```python
from build123d import *

# Parameters (mm, degrees)
SKETCH1_R           = 1.5
BOSS_EXTRUDE1_DEPTH = 5
SKETCH2_W           = 10
SKETCH2_H           = 5
CUT_EXTRUDE1_DEPTH  = 5


with BuildPart() as part:
    # Sketch1 → Boss-Extrude1 (new body)
    with BuildSketch(Plane(origin=(0, 0, 0), x_dir=(0, 0, -1), z_dir=(1, 0, 0))):
        with BuildLine():
            Line((-10, 15), (-30, 15))
            Line((-30, 15), (-30, -10))
            Line((-30, -10), (0, -10))
            ThreePointArc((0, -10), (7.071067812, -7.071067812), (10, 0))
            Line((10, 0), (10, 50))
            ThreePointArc((10, 50), (0, 60), (-10, 50))
            Line((-10, 50), (-10, 15))
        make_face()
        with Locations((0, 50)):
            Circle(SKETCH1_R, mode=Mode.SUBTRACT)
        Circle(SKETCH1_R, mode=Mode.SUBTRACT)
    extrude(amount=BOSS_EXTRUDE1_DEPTH)

    # Sketch2 → Cut-Extrude1 (cut)
    with BuildSketch(Plane(origin=(5, 0, 0), x_dir=(0, 0, -1), z_dir=(1, 0, 0))):
        with Locations((-25, 7.5)):
            Rectangle(SKETCH2_W, SKETCH2_H)
        with Locations((-25, -2.5)):
            Rectangle(SKETCH2_W, SKETCH2_H)
    extrude(amount=-CUT_EXTRUDE1_DEPTH, mode=Mode.SUBTRACT)


solid = part.part
```
Check sheet for the modelled part. Datum: model origin and axes. Units: mm. A direction names the side the tool comes from. Round coordinates to 2 decimals unless told otherwise and drop trailing zeros. Order: outer loops, then holes, each group sorted by start corner. A loop starts at its lowest first (then second) coordinate and runs counter-clockwise, first axis right, second up. Notation, with made-up numbers: (1.25, -13) -> (43.25, -13) arc R24 ccw to (43.25, 13) -> close; hole circle Ø2 at (32.25, -36). An arc over 180 degrees is marked (long way). Use CSV: the item, a comma, the result in double quotes.
(1) Draft check along Z on faces 1 (the face through (2.46, 0.07, 1.5)), 2 (the face through (2, -10, 15)), 3 (the face through (2, 13, 30)), 4 (the face through (2, 60, 0)). Enter one of: pulls with the +Z half, pulls with the -Z half, needs draft (parallel to the pull), parting line crosses it, or undercut.
Worked out:
face 1,"undercut"
face 2,"needs draft"
face 3,"pulls with the +Z half"
face 4,"parting line crosses it"
(2) Depth check by flat-ended pin: pin 1 (1.5 mm diameter, centred on x = 3.5, y = -3.5, fed in from +Z); pin 2 (1.5 mm diameter, centred on x = 2, z = 26.5, fed in from +Y); pin 3 (1.5 mm diameter, centred on x = 2.5, y = 35.5, fed in from +Z); pin 4 (2.5 mm diameter, centred on y = 0, z = 0, fed in from -X). Enter the tip coordinate at first touch or a pass-through.
Worked out:
pin 1,"z = 20"
pin 2,"y = 15"
pin 3,"z = 10"
pin 4,"through"
(3) Cross-section at B-B (z = 12). Record the boundary of the cut face in (x, y), and give its area (3 significant figures).
Worked out:
outline,"(0, -10) -> (5, -10) -> (5, 15) -> (0, 15) -> close"
area,"125 mm²"
(4) Material ranges on line 1 along Y through (x, z) = (1.75, 0); line 2 along Z through (x, y) = (3.85, 8); line 3 along Z through (x, y) = (0.5, 43), recorded low to high. Write a range as from..to.
Worked out:
line 1,"-10..-1.5, 1.5..48.5, 51.5..60"
line 2,"-10..20"
line 3,"-10..10"
(5) Cross-section at A-A (x = 1.45). Record the boundary of the cut face in (y, z).
Worked out:
outline,"(-10, 0) arc R10 ccw to (0, -10) -> (50, -10) arc R10 ccw to (50, 10) -> (15, 10) -> (15, 30) -> (10, 30) -> (10, 20) -> (5, 20) -> (5, 30) -> (0, 30) -> (0, 20) -> (-5, 20) -> (-5, 30) -> (-10, 30) -> close; hole circle Ø3 at (0, 0); hole circle Ø3 at (50, 0)"
(6) Tool access check on faces 5 (the face through (2, 15, 20)), 6 (the face through (5, 18, 6)), 7 (the face through (3, 7, 20)). Record the directions out of +Z, -Z, +X, -X, +Y, -Y that give a thin tool (end or side, any length) a straight path to the whole face; none if there is none.
Worked out:
face 5,"+Z, +X, -X, +Y"
face 6,"+Z, -Z, +X, +Y, -Y"
face 7,"+Z, +X, -X"
(7) Cross-section at C-C (y = 26.5). Record the boundary of the cut face in (x, z).
Worked out:
outline,"(0, -10) -> (5, -10) -> (5, 10) -> (0, 10) -> close"
